from build123d import *

# Parameters (mm, degrees)
F0_R     = 1.5
F0_W     = 0.5
F0_H     = 3.5
F0_H_2   = 0.5
F1_DEPTH = 1
F2_DEPTH = 5
F3_DEPTH = 2
F4_DEPTH = 4
F5_R     = 0.75
F6_DEPTH = 25


with BuildPart() as f1:
    # F0 (on Top) → F1 (new body)
    with BuildSketch(Plane.XY):
        with BuildLine():
            Line((2, -3.5), (2, 0))
            Line((2, 0), (2, 3.5))
            Line((2, 3.5), (-6.5766632877, 3.5))
            ThreePointArc((-6.5766632877, 3.5), (-7.45, 0), (-6.5766632877, -3.5))
            Line((-6.5766632877, -3.5), (2, -3.5))
        make_face()
        Circle(F0_R, mode=Mode.SUBTRACT)
        with Locations((2.25, -1.75)):
            Rectangle(F0_W, F0_H)
        with Locations((2.25, 1.75)):
            Rectangle(F0_W, F0_H)
        with BuildLine():
            ThreePointArc((-6.2851014312, -4), (-6.4357398892, -3.7528325408), (-6.5766632877, -3.5))
            Line((-6.5766632877, -3.5), (-7.1381019886, -3.5))
            ThreePointArc((-7.1381019886, -3.5), (-7.0087149266, -3.7523879167), (-6.8704075571, -4))
            Line((-6.8704075571, -4), (-6.2851014312, -4))
        make_face()
        with BuildLine():
            Line((-7.1381019886, 3.5), (-6.5766632877, 3.5))
            ThreePointArc((-6.5766632877, 3.5), (-6.4357398892, 3.7528325408), (-6.2851014312, 4))
            Line((-6.2851014312, 4), (-6.8704075571, 4))
            ThreePointArc((-6.8704075571, 4), (-7.0087149266, 3.7523879167), (-7.1381019886, 3.5))
        make_face()
        with Locations((2.25, 3.75)):
            Rectangle(F0_W, F0_H_2)
        with Locations((2.25, -3.75)):
            Rectangle(F0_W, F0_H_2)
        with BuildLine():
            ThreePointArc((-6.5766632877, -3.5), (-7.45, 0), (-6.5766632877, 3.5))
            Line((-6.5766632877, 3.5), (-7.1381019886, 3.5))
            ThreePointArc((-7.1381019886, 3.5), (-7.95, 0), (-7.1381019886, -3.5))
            Line((-7.1381019886, -3.5), (-6.5766632877, -3.5))
        make_face()
        with BuildLine():
            Line((-6.5766632877, 3.5), (2, 3.5))
            Line((2, 3.5), (2, 4))
            Line((2, 4), (-6.2851014312, 4))
            ThreePointArc((-6.2851014312, 4), (-6.4357398892, 3.7528325408), (-6.5766632877, 3.5))
        make_face()
        with BuildLine():
            Line((2, -4), (2, -3.5))
            Line((2, -3.5), (-6.5766632877, -3.5))
            ThreePointArc((-6.5766632877, -3.5), (-6.4357398892, -3.7528325408), (-6.2851014312, -4))
            Line((-6.2851014312, -4), (2, -4))
        make_face()
    extrude(amount=F1_DEPTH)

    # F0 (on Top) → F2 (join)
    with BuildSketch(Plane.XY):
        with Locations((2.25, -1.75)):
            Rectangle(F0_W, F0_H)
        with Locations((2.25, 1.75)):
            Rectangle(F0_W, F0_H)
        with BuildLine():
            ThreePointArc((-6.2851014312, -4), (-6.4357398892, -3.7528325408), (-6.5766632877, -3.5))
            Line((-6.5766632877, -3.5), (-7.1381019886, -3.5))
            ThreePointArc((-7.1381019886, -3.5), (-7.0087149266, -3.7523879167), (-6.8704075571, -4))
            Line((-6.8704075571, -4), (-6.2851014312, -4))
        make_face()
        with Locations((2.25, -3.75)):
            Rectangle(F0_W, F0_H_2)
        with Locations((2.25, 3.75)):
            Rectangle(F0_W, F0_H_2)
        with BuildLine():
            Line((-7.1381019886, 3.5), (-6.5766632877, 3.5))
            ThreePointArc((-6.5766632877, 3.5), (-6.4357398892, 3.7528325408), (-6.2851014312, 4))
            Line((-6.2851014312, 4), (-6.8704075571, 4))
            ThreePointArc((-6.8704075571, 4), (-7.0087149266, 3.7523879167), (-7.1381019886, 3.5))
        make_face()
        with BuildLine():
            ThreePointArc((-6.5766632877, -3.5), (-7.45, 0), (-6.5766632877, 3.5))
            Line((-6.5766632877, 3.5), (-7.1381019886, 3.5))
            ThreePointArc((-7.1381019886, 3.5), (-7.95, 0), (-7.1381019886, -3.5))
            Line((-7.1381019886, -3.5), (-6.5766632877, -3.5))
        make_face()
    extrude(amount=F2_DEPTH)

    # F0 (on Top) → F3 (join)
    with BuildSketch(Plane.XY):
        with BuildLine():
            Line((2, -4), (2, -3.5))
            Line((2, -3.5), (-6.5766632877, -3.5))
            ThreePointArc((-6.5766632877, -3.5), (-6.4357398892, -3.7528325408), (-6.2851014312, -4))
            Line((-6.2851014312, -4), (2, -4))
        make_face()
        with BuildLine():
            Line((-6.5766632877, 3.5), (2, 3.5))
            Line((2, 3.5), (2, 4))
            Line((2, 4), (-6.2851014312, 4))
            ThreePointArc((-6.2851014312, 4), (-6.4357398892, 3.7528325408), (-6.5766632877, 3.5))
        make_face()
    extrude(amount=F3_DEPTH)

    # F4 (add): a face of the model
    f4_faces = [f1.faces().sort_by_distance(p)[0] for p in [
        (-7.5317140669, 0, 5),
    ]]
    extrude(f4_faces, amount=F4_DEPTH)

    # F5 (on Right) → F6 (cut)
    with BuildSketch(Plane.YZ):
        with BuildLine():
            ThreePointArc((2.75, 4), (2, 4.75), (1.25, 4))
            ThreePointArc((1.25, 4), (2, 3.25), (2.75, 4))
        make_face()
        with BuildLine():
            Line((0, 4), (0, 3.25))
            ThreePointArc((0, 3.25), (0.5303300859, 3.4696699141), (0.75, 4))
            Line((0.75, 4), (0, 4))
        make_face()
        with BuildLine():
            Line((0, 4.75), (0, 4))
            Line((0, 4), (0.75, 4))
            ThreePointArc((0.75, 4), (0.5303300859, 4.5303300859), (0, 4.75))
        make_face()
        with BuildLine():
            ThreePointArc((-0.75, 4), (-0.5303300859, 3.4696699141), (0, 3.25))
            Line((0, 3.25), (0, 4))
            Line((0, 4), (-0.75, 4))
        make_face()
        with Locations((-2, 4)):
            Circle(F5_R)
        with BuildLine():
            Line((-0.75, 4), (0, 4))
            Line((0, 4), (0, 4.75))
            ThreePointArc((0, 4.75), (-0.5303300859, 4.5303300859), (-0.75, 4))
        make_face()
        with Locations((2, 7.5)):
            Circle(F5_R)
        with Locations((0, 7.5)):
            Circle(F5_R)
        with Locations((-2, 7.5)):
            Circle(F5_R)
    extrude(amount=-F6_DEPTH, mode=Mode.SUBTRACT)


solid = f1.part
Can you work these out from the model? Positions are in its coordinate system, mm. A direction names the side the tool comes from. Round coordinates to 2 decimals unless told otherwise and drop trailing zeros. Order: outer loops, then holes, each group sorted by start corner. A loop starts at its lowest first (then second) coordinate and runs counter-clockwise, first axis right, second up. Notation, with made-up numbers: M -15,-27 L -10,-27 A26 cw -10,0 Z; hole C -4,43.5 d11. An arc over 180 degrees is marked long. Use a Markdown table: item, result.
1) If I drill on line 1 along Z through (x, y) = (-7.5, 2); line 2 along Y through (x, z) = (-1.5, 1.5); line 3 along Y through (x, z) = (-7.6, 7.5), over which ranges is the centre line in solid material (lowest first)?
Geometry says:
| item | result |
|---|---|
| line 1 | z = 0 to 3.25, 4.75 to 6.75, 8.25 to 9 |
| line 2 | y = -4 to -3.5, 3.5 to 4 |
| line 3 | y = -1.25 to -0.75, 0.75 to 1.25 |
2) If we mould it in two halves opening along X, with no side actions, what happens to faces 4 (the face through (-2.6, -4, 1.8)), 5 (the face through (-3, 0, 1)), 6 (the face through (2.5, 0, 2))? For each: +X half, -X half, draft (parallel to the pull), parting line (faces both ways), or undercut.
Geometry says:
| item | result |
|---|---|
| face 4 | draft |
| face 5 | undercut |
| face 6 | +X half |
3) Imagine slicing it at A-A (x = 0). List the corners of the cut face in (y, z) for me, then the cut area to 3 significant figures.
Geometry says:
| item | result |
|---|---|
| outline | M -4,0 L -1.5,0 L -1.5,1 L -3.5,1 L -3.5,2 L -4,2 Z; M 1.5,0 L 4,0 L 4,2 L 3.5,2 L 3.5,1 L 1.5,1 Z |
| area | 6.00 mm² |
4) Imagine slicing it at D-D (x = -4.5). List the corners of the cut face in (y, z) for me, then the cut area to 3 significant figures.
Geometry says:
| item | result |
|---|---|
| outline | M -4,0 L 4,0 L 4,2 L 3.5,2 L 3.5,1 L -3.5,1 L -3.5,2 L -4,2 Z |
| area | 9.00 mm² |
5) Imagine slicing it at C-C (z = 7.5). List the corners of the cut face in (x, y) for me, then the cut area to 3 significant figures.
Geometry says:
| item | result |
|---|---|
| outline | M -7.91,-0.75 A7.95 ccw -7.85,-1.25 L -7.34,-1.25 A7.45 cw -7.41,-0.75 Z; M -7.91,0.75 L -7.41,0.75 A7.45 cw -7.34,1.25 L -7.85,1.25 A7.95 ccw Z; M -7.46,-2.75 A7.95 ccw -6.87,-4 L -6.29,-4 A7.45 cw -6.92,-2.75 Z; M -7.46,2.75 L -6.92,2.75 A7.45 cw -6.29,4 L -6.87,4 A7.95 ccw Z |
| area | 1.90 mm² |
6) On a 3-axis mill with a long thin cutter (end or side, diameter ignored), from which of +Z, -Z, +X, -X, +Y, -Y can I reach the whole of each face in a straight line? I mean faces 1 (the face through (-7.6, 0.3, 9)), 2 (the face through (-7.381, -2.163, 3.268)), 3 (the face through (-2.2, -3.5, 1.5)). Say none if no direction works.
Geometry says:
| item | result |
|---|---|
| face 1 | +Z, +X, -X, +Y, -Y |
| face 2 | -X |
| face 3 | +Z |
7) I'm going to push flat-ended pins straight in: P1, Ø0.6, axis at x = 2.5, y = 1, coming from the +Z side; P2, Ø2, axis at x = -4, y = -0.5, coming from the +Z side; P3, Ø2, axis at y = 2.5, z = 4, coming from the -X side. Where does each tip first touch, or does it pass through?
Geometry says:
| item | result |
|---|---|
| P1 | stops at z = 5 |
| P2 | stops at z = 1 |
| P3 | stops at x = -7.74 |
8) Imagine slicing it at B-B (y = 2.5). List the corners of the cut face in (x, z) for me, then the cut area to 3 significant figures.
Geometry says:
| item | result |
|---|---|
| outline | M -7.55,0 L 2.5,0 L 2.5,5 L 2,5 L 2,1 L -7.02,1 L -7.02,3.44 L -7.55,3.44 Z; M -7.55,4.56 L -7.02,4.56 L -7.02,6.94 L -7.55,6.94 Z; M -7.55,8.06 L -7.02,8.06 L -7.02,9 L -7.55,9 Z |
| area | 15.1 mm² |
